```python
from build123d import *

# Parameters (mm, degrees)
F0_W     = 273.05
F0_H     = 114.3
F0_R     = 38.1
F1_DEPTH = 25.4
F3_DEPTH = 25.4
F5_DEPTH = 25.4


with BuildPart() as f1:
    # F0 (on Front) → F1 (new body)
    with BuildSketch(Plane.XZ):
        with Locations((136.525, 57.15)):
            Rectangle(F0_W, F0_H)
        with Locations((47.625, 57.15)):
            Circle(F0_R, mode=Mode.SUBTRACT)
        with Locations((225.425, 57.15)):
            Circle(F0_R, mode=Mode.SUBTRACT)
    extrude(amount=F1_DEPTH)

    # F2 (on face) → F3 (cut)
    with BuildSketch(Plane.XZ.offset(25.4)):
        with BuildLine():
            Line((177.8, 114.3), (95.25, 114.3))
            Line((95.25, 114.3), (95.25, 49.53))
            ThreePointArc((95.25, 49.53), (98.597769, 41.447769), (106.68, 38.1))
            Line((106.68, 38.1), (166.37, 38.1))
            ThreePointArc((166.37, 38.1), (174.452231, 41.447769), (177.8, 49.53))
            Line((177.8, 49.53), (177.8, 114.3))
        make_face()
    extrude(amount=-F3_DEPTH, mode=Mode.SUBTRACT)

    # F4 (on face) → F5 (cut)
    with BuildSketch(Plane.XZ.offset(25.4)):
        Polygon((166.37, 30.481706), (166.37, 38.1), (145.37774, 38.1), (145.37774, 30.481706), (74.835515, 30.481706), (47.264424, 19.051706), (225.064424, 19.051706), (198.214485, 30.481706), align=None)
    extrude(amount=-F5_DEPTH, mode=Mode.SUBTRACT)


solid = f1.part
```
The listing builds one solid part. Answer for the finished solid, in the listing's coordinates (mm). A direction names the side the tool comes from. Give positions to 0.01 mm unless a question says otherwise; leave off trailing zeros. Write each loop counter-clockwise with the first axis right and the second up, starting at its lowest first coordinate (ties: lowest second). Pieces come first, ordered by that corner, then holes. Notation, with made-up numbers: M 56,8.25 L 86,8.25 A37 ccw 86,44.25 Z; hole C 60.5,37.25 d6. An arc over 180 degrees is marked long. Write each question's results on one line, items separated by ' | '.
Q1. A flat-ended cylindrical pin translates along its axis: P1, Ø7.5, axis at x = 187, y = -13, coming from the -Z side. Find the tip coordinate at first contact, or state that the pin passes through.
Output values:
P1: z = 0
Q2. Section B-B, the plane z = 104 is taken. Write down the section's boundary in (x, y).
Output values:
outline: M 0,-25.4 L 95.25,-25.4 L 95.25,0 L 0,0 Z; M 177.8,-25.4 L 273.05,-25.4 L 273.05,0 L 177.8,0 Z
Q3. A tool of negligible diameter and unlimited length cuts with its end or side. For faces 4 (the flat face through (166.37, -13, 34)), 5 (the flat face through (225, -13, 114.3)), 6 (the flat face through (135, -13, 19.052)), from which of +Z, -Z, +X, -X, +Y, -Y can it reach the whole face along a straight path? Write none if from no direction.
Output values:
face 4: +Z, +Y, -Y | face 5: +Z, +X, -X, +Y, -Y | face 6: +Y, -Y
Q4. For a pull along X with two mould halves and no side action, classify faces 1 (the flat face through (126, -13, 38.1)), 2 (the flat face through (0, -13, 56)), 3 (the flat face through (273.05, -13, 56)) as released by +X, released by -X, zero draft, split by the parting line, or undercut.
Output values:
face 1: undercut | face 2: released by -X | face 3: released by +X
Q5. Section A-A, the plane x = 116 is taken. Write down the section's boundary in (y, z).
Output values:
outline: M -25.4,0 L 0,0 L 0,19.05 L -25.4,19.05 Z; M -25.4,30.48 L 0,30.48 L 0,38.1 L -25.4,38.1 Z
Q6. Section D-D, the plane z = 57.15 is taken. Write down the section's boundary in (x, y) (3 decimals), then the cut area to 3 significant figures.
Output values:
outline: M 0,-25.4 L 9.525,-25.4 L 9.525,0 L 0,0 Z; M 85.725,-25.4 L 95.25,-25.4 L 95.25,0 L 85.725,0 Z; M 177.8,-25.4 L 187.325,-25.4 L 187.325,0 L 177.8,0 Z; M 263.525,-25.4 L 273.05,-25.4 L 273.05,0 L 263.525,0 Z | area: 968 mm2
Q7. Consider L1, parallel to X at y = -18, z = 57.15 (3 decimals); L2, parallel to Z at x = 179, y = -5.5; L3, parallel to X at y = -6, z = 83.5. Determine where each line is inside the solid, lowest interval first. Write a range as from..to.
Output values:
L1: 0..9.525, 85.725..95.25, 177.8..187.325, 263.525..273.05 | L2: 0..19.05, 30.48..114.3 | L3: 0..20.11, 75.14..95.25, 177.8..197.91, 252.94..273.05
Q8. Section C-C, the plane y = -21 is taken. Write down the section's boundary in (x, z) (3 decimals).
Output values:
outline: M 0,0 L 273.05,0 L 273.05,114.3 L 177.8,114.3 L 177.8,49.53 A11.43 cw 166.37,38.1 L 166.37,30.482 L 198.214,30.482 A38.1 cw long 225.064,19.052 L 47.986,19.052 A38.1 cw long 74.836,30.482 L 145.378,30.482 L 145.378,38.1 L 106.68,38.1 A11.43 cw 95.25,49.53 L 95.25,114.3 L 0,114.3 Z
